Can you work these out from the drawing? Everything is in mm from the part's minimum corner. Coordinates: 2 decimals unless noted, no trailing zeros. Loops run counter-clockwise (first coordinate to the right, second up) from the corner with the lowest first, then second, coordinate; pieces in that order, holes last. Notation, with made-up numbers: (-30.5, -12) - (-9.5, -12) arc R34 cw to (-9.5, 26) - close; hole circle Ø11 at (59, -12.5). An arc over 180 degrees is marked (long way). Use CSV: the item, a comma, the result in double quotes.
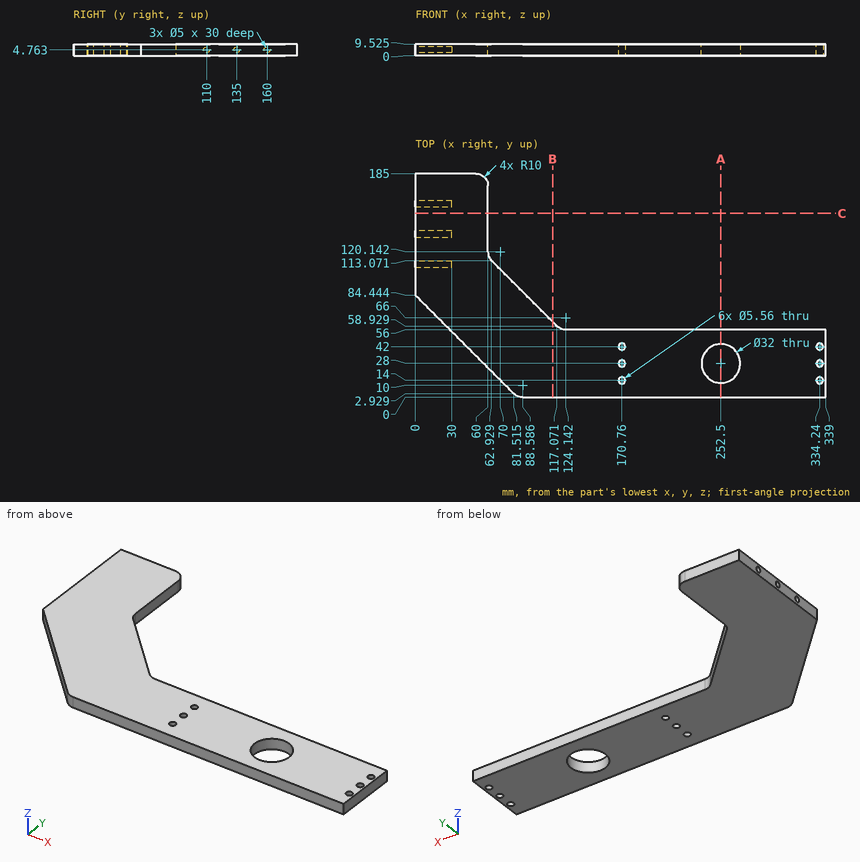
(1) Please list where these lines run through material, in increasing order: line 1 (Z direction, x = 19.75, y = 160) (1 decimal); line 2 (Y direction, x = 334.24, z = 3.75); line 3 (Y direction, x = 25, z = 3) (1 decimal).
Computed:
line 1,"z = 0 to 2.3, 7.3 to 9.5"
line 2,"y = 0 to 11.22, 16.78 to 25.22, 30.78 to 39.22, 44.78 to 56"
line 3,"y = 59.4 to 108.2, 111.8 to 133.2, 136.8 to 158.2, 161.8 to 185"
(2) Suppose I cut it at A-A (x = 252.5). Write out the boundary of the cut face in (y, z) (1 decimal).
Computed:
outline,"(0, 0) - (12, 0) - (12, 9.5) - (0, 9.5) - close; (44, 0) - (56, 0) - (56, 9.5) - (44, 9.5) - close"
(3) Suppose I cut it at C-C (y = 152). Write out the boundary of the cut face in (x, z) (1 decimal).
Computed:
outline,"(0, 0) - (60, 0) - (60, 9.5) - (0, 9.5) - close"
(4) Suppose I cut it at B-B (x = 113.5). Write out the boundary of the cut face in (y, z) (1 decimal), plus the area to 3 significant figures.
Computed:
outline,"(0, 0) - (62.5, 0) - (62.5, 9.5) - (0, 9.5) - close"
area,"595 mm²"
(5) Will these pins go through, and if not, where does the flat tip stop? pin 1 (2 mm diameter, centred on x = 236.5, z = 2.5, fed in from -Y); pin 2 (1.5 mm diameter, centred on y = 110.5, z = 5.5, fed in from -X); pin 3 (2 mm diameter, centred on x = 79.5, z = 5.5, fed in from -Y) (1 decimal); pin 4 (3 mm diameter, centred on y = 110, z = 4.76, fed in from +X).
Computed:
pin 1,"stops at y = 0"
pin 2,"stops at x = 30"
pin 3,"stops at y = 3.9"
pin 4,"stops at x = 67.5"
